Part model, mm, in its own coordinate system. A direction names the side the tool comes from. Round coordinates to 2 decimals unless told otherwise and drop trailing zeros. Loops run counter-clockwise (first coordinate to the right, second up) from the corner with the lowest first, then second, coordinate; pieces in that order, holes last.
(1) Cut at D-D on y = -2.5. List the corners of the cut face in (x, z) (3 decimals).
(2) Tool access for faces 4 (the face through (22, 0, 15.875)), 5 (the face through (5, -12.7, 8)), 6 (the face through (17, 12.7, 8)), 7 (the face through (9.525, -3, 16.2)), 8 (the face through (12.7, -10, 8)): list every direction of +Z, -Z, +X, -X, +Y, -Y with a clear straight run to the whole face (end or side of a thin tool).
(3) Cut at C-C on x = 10. List the corners of the cut face in (y, z) (3 decimals).
(4) Cut at B-B on y = -8. List the corners of the cut face in (x, z) (3 decimals), then the cut area to 3 significant figures.
(5) Probe probe 1 along X at (y, z) = (-7.25, 9.25) (3 decimals); probe 2 along Z at (x, y) = (27.5, -1.25) (3 decimals); probe 3 along X at (y, z) = (-6.5, 20.25) (3 decimals). List the from-to ranges inside material, lowest first.
(6) Cut at A-A on z = 10.75. List the corners of the cut face in (x, y) (3 decimals), then the cut area to 3 significant figures.
(7) Flat gauge pins, fed straight in: pin 1 (1.9 mm diameter, centred on y = -9, z = 9.5, fed in from -X); pin 2 (1 mm diameter, centred on x = 11.5, z = 5.5, fed in from -Y); pin 3 (1.5 mm diameter, centred on x = 18.5, y = 1.5, fed in from +Z) (3 decimals). Where does each tip first touch, or does it go through?
(8) Mould opens along X. For faces 1 (the face through (5, 0, 22.225)), 2 (the face through (11, -6.35, 8)), 3 (the face through (0, 0, 11)) say: +X half, -X half, draft (parallel to the pull), parting line (faces both ways), or undercut.
from build123d import *

# Parameters (mm, degrees)
F0_W     = 34.925
F0_H     = 22.225
F1_DEPTH = 12.7
F3_DEPTH = 34.926
F5_DEPTH = 25.4
F7_DEPTH = 34.926
F8_W     = 3.175
F8_H     = 6.35
F9_DEPTH = 15.876


with BuildPart() as f1:
    # F0 (on Front) → F1 (new body, symmetric)
    with BuildSketch(Plane.XZ):
        with Locations((17.4625, 11.1125)):
            Rectangle(F0_W, F0_H)
    extrude(amount=F1_DEPTH, both=True)

    # F2 (on face) → F3 (cut, through all)
    with BuildSketch(Plane(origin=(0, 0, 0), x_dir=(0, -1, 0), z_dir=(-1, 0, 0))):
        Polygon((12.7, 15.875), (12.7, 22.225), (6.35, 22.225), align=None)
    extrude(amount=-F3_DEPTH, mode=Mode.SUBTRACT)

    # F4 (on face) → F5 (cut)
    with BuildSketch(Plane.YZ.offset(34.925)):
        Polygon((-6.35, 22.225), (-12.7, 15.875), (12.7, 15.875), (12.7, 22.225), align=None)
    extrude(amount=-F5_DEPTH, mode=Mode.SUBTRACT)

    # F6 (on face) → F7 (cut, through all)
    with BuildSketch(Plane(origin=(0, 0, 0), x_dir=(0, -1, 0), z_dir=(-1, 0, 0))):
        Polygon((-6.35, 22.225), (-12.7, 22.225), (-12.7, 15.875), align=None)
    extrude(amount=-F7_DEPTH, mode=Mode.SUBTRACT)

    # F8 (on face) → F9 (cut, through all)
    with BuildSketch(Plane.XY.offset(15.875)):
        with Locations((11.1125, -9.525)):
            Rectangle(F8_W, F8_H)
    extrude(amount=-F9_DEPTH, mode=Mode.SUBTRACT)


solid = f1.part
Final values:
1. outline: (0, 0) - (34.925, 0) - (34.925, 15.875) - (9.525, 15.875) - (9.525, 22.225) - (0, 22.225) - close
2. face 4: +Z, +X, +Y, -Y
2. face 5: +Z, -Z, +X, -X, -Y
2. face 6: +Z, -Z, +X, -X, +Y
2. face 7: +Z, -Y
2. face 8: +Z, -Z, -Y
3. outline: (-6.35, 0) - (12.7, 0) - (12.7, 15.875) - (-6.35, 15.875) - close
4. outline: (0, 0) - (9.525, 0) - (9.525, 20.575) - (0, 20.575) - close; (12.7, 0) - (34.925, 0) - (34.925, 15.875) - (12.7, 15.875) - close
4. area: 549 mm2
5. probe 1: x = 0 to 9.525, 12.7 to 34.925
5. probe 2: z = 0 to 15.875
5. probe 3: x = 0 to 9.525
6. outline: (0, -12.7) - (9.525, -12.7) - (9.525, -6.35) - (12.7, -6.35) - (12.7, -12.7) - (34.925, -12.7) - (34.925, 12.7) - (0, 12.7) - close
6. area: 867 mm2
7. pin 1: stops at x = 0
7. pin 2: stops at y = -6.35
7. pin 3: stops at z = 15.875
8. face 1: draft
8. face 2: undercut
8. face 3: -X half
